Source: CAD feature listing. Evaluate the final solid. Frame: model axes, mm. Give positions to 0.01 mm unless a question says otherwise; leave off trailing zeros. Write each loop counter-clockwise with the first axis right and the second up, starting at its lowest first coordinate (ties: lowest second). Pieces come first, ordered by that corner, then holes. Notation, with made-up numbers: M 72.25,22 L 118.25,22 A9 cw 118.25,26 Z; hole C 25,89 d8. An arc over 180 degrees is marked long. Return JSON: item names as keys, results as strings.
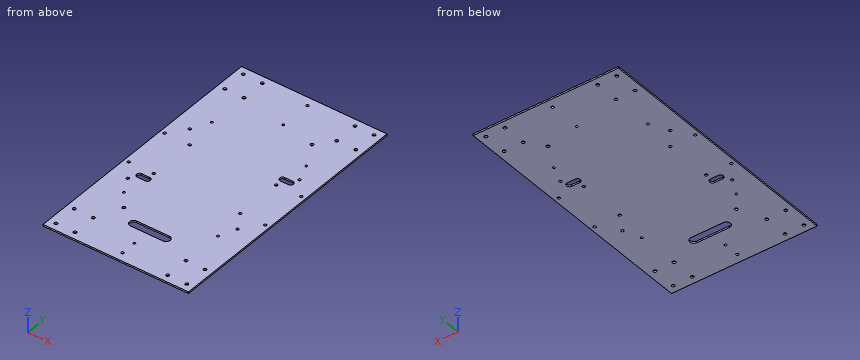
```python
from build123d import *

# Parameters (mm, degrees)
CROQUIS1_W                     = 179
CROQUIS1_H                     = 320
SALIENTE_EXTRUIR1_DEPTH        = 2
TALADRO_DE_MARGEN_PARA_M31_D   = 3.4
TALADRO_DE_MARGEN_PARA_M2_51_D = 2.9
TALADRO_DE_MARGEN_PARA_M32_D   = 3.4
CORTAR_EXTRUIR1_DEPTH          = 184.34189374
TALADRO_DE_MARGEN_PARA_M3_51_D = 3.9
SIMETR_A4_COPY_1_D             = 3.9
TALADRO_DE_MARGEN_PARA_M3_52_D = 3.9
CORTAR_EXTRUIR2_DEPTH          = 184.34189374


with BuildPart() as part:
    # Croquis1 → Saliente-Extruir1 (new body)
    with BuildSketch(Plane.XY):
        Rectangle(CROQUIS1_W, CROQUIS1_H)
    extrude(amount=SALIENTE_EXTRUIR1_DEPTH)

    # Taladro de margen para M31 (through all)
    with Locations(Plane.XY.offset(2)):
        with Locations((0, 149), (-68.69, 49.42), (-68.69, -50.58), (0, -149), (66.31, -50.58), (66.31, 49.42)):
            Hole(TALADRO_DE_MARGEN_PARA_M31_D / 2)

    # Taladro de margen para M2.51 (through all)
    with Locations(Plane.XY.offset(2)):
        with Locations((0, 110), (-58, 71), (-58, -71), (0, -130), (58, -71), (58, 71)):
            Hole(TALADRO_DE_MARGEN_PARA_M2_51_D / 2)

    # Taladro de margen para M32 (through all)
    with Locations(Plane.XY.offset(2)):
        with Locations((-84, 29), (-84, -29), (-53.252582689, 29), (-53.252582689, -29), (53.252582689, 29), (84, 29), (84, -29), (53.252582689, -29)):
            Hole(TALADRO_DE_MARGEN_PARA_M32_D / 2)

    # Croquis10 → Cortar-Extruir1 (cut, through all)
    with BuildSketch(Plane.XY.offset(2)):
        with BuildLine():
            Line((-62.5, -36.5), (-52.5, -36.5))
            ThreePointArc((-52.5, -36.5), (-49, -40), (-52.5, -43.5))
            Line((-52.5, -43.5), (-62.5, -43.5))
            ThreePointArc((-62.5, -43.5), (-66, -40), (-62.5, -36.5))
        make_face()
        with BuildLine():
            Line((52.5, 43.5), (62.5, 43.5))
            ThreePointArc((62.5, 43.5), (66, 40), (62.5, 36.5))
            Line((62.5, 36.5), (52.5, 36.5))
            ThreePointArc((52.5, 36.5), (49, 40), (52.5, 43.5))
        make_face()
    extrude(amount=-CORTAR_EXTRUIR1_DEPTH, mode=Mode.SUBTRACT)

    # Taladro de margen para M3.51 (through all)
    with Locations(Plane.XY.offset(2)):
        with Locations((-80.5, -121.42), (-57, -121.42), (-57, -151), (-80.5, -151)):
            taladro_de_margen_para_m3_51 = Hole(TALADRO_DE_MARGEN_PARA_M3_51_D / 2)

    # Simetría3: Taladro de margen para M3.51 across plane
    add(taladro_de_margen_para_m3_51.mirror(Plane.ZX), mode=Mode.SUBTRACT)

    # Simetría4: Taladro de margen para M3.51 across plane
    add(taladro_de_margen_para_m3_51.mirror(Plane(origin=(0, 0, 0), x_dir=(0, 0, 1), z_dir=(1, 0, 0))), mode=Mode.SUBTRACT)

    # Simetría4 copy 1 (through all)
    with Locations(Plane(origin=(0, 0, 2), x_dir=(-1, 0, 0), z_dir=(0, 0, 1))):
        with Locations((-80.5, -121.42), (-57, -121.42), (-57, -151), (-80.5, -151)):
            Hole(SIMETR_A4_COPY_1_D / 2)

    # Taladro de margen para M3.52 (through all)
    with Locations(Plane(origin=(0, 0, 0), x_dir=(-1, 0, 0), z_dir=(0, 0, -1))):
        with Locations((-41.6, 101.784994015), (43.2, -90.415005985)):
            Hole(TALADRO_DE_MARGEN_PARA_M3_52_D / 2)

    # Croquis17 → Cortar-Extruir2 (cut, through all)
    with BuildSketch(Plane(origin=(0, 0, 0), x_dir=(-1, 0, 0), z_dir=(0, 0, -1))):
        with BuildLine():
            Line((20, -110), (-20, -110))
            ThreePointArc((-20, -110), (-25, -105), (-20, -100))
            Line((-20, -100), (20, -100))
            ThreePointArc((20, -100), (25, -105), (20, -110))
        make_face()
    extrude(amount=-CORTAR_EXTRUIR2_DEPTH, mode=Mode.SUBTRACT)


solid = part.part
```
1) Cut plane C-C, the plane z = 1. Give the number of separate pieces and of enclosed holes in the cut face, then the cut area to 3 significant figures.
Numbers:
{"separate pieces": "1", "enclosed holes": "41", "area": "56,200 mm²"}
2) Line query: line 1 (Y direction, x = 84, z = 1.3); line 2 (Y direction, x = -80.5, z = 1); line 3 (Y direction, x = 81, z = 0.65). Output: solid intervals per line, ascending. Write a range as [from, to].
Numbers:
{"line 1": "y = [-160, -30.7], [-27.3, 27.3], [30.7, 160]", "line 2": "y = [-160, -152.95], [-149.05, -123.37], [-119.47, 119.47], [123.37, 149.05], [152.95, 160]", "line 3": "y = [-160, -152.88], [-149.12, -123.3], [-119.54, 119.54], [123.3, 149.12], [152.88, 160]"}
3) Contact query for a flat-ended pin moving along its axis: pin 1 Ø3 at (x, y) = (41.6, 101.78) entering from +Z (1 decimal). Output: stop coordinate, or through.
Numbers:
{"pin 1": "passes through"}
4) Cut plane A-A, the plane y = 40. Return the cut outline in (x, z), then the cut area to 3 significant figures.
Numbers:
{"outline": "M -89.5,0 L 49,0 L 49,2 L -89.5,2 Z; M 66,0 L 89.5,0 L 89.5,2 L 66,2 Z", "area": "324 mm²"}
5) Cut plane B-B, the plane x = -17. Return the cut outline in (y, z).
Numbers:
{"outline": "M -160,0 L -110,0 L -110,2 L -160,2 Z; M -100,0 L 160,0 L 160,2 L -100,2 Z"}
